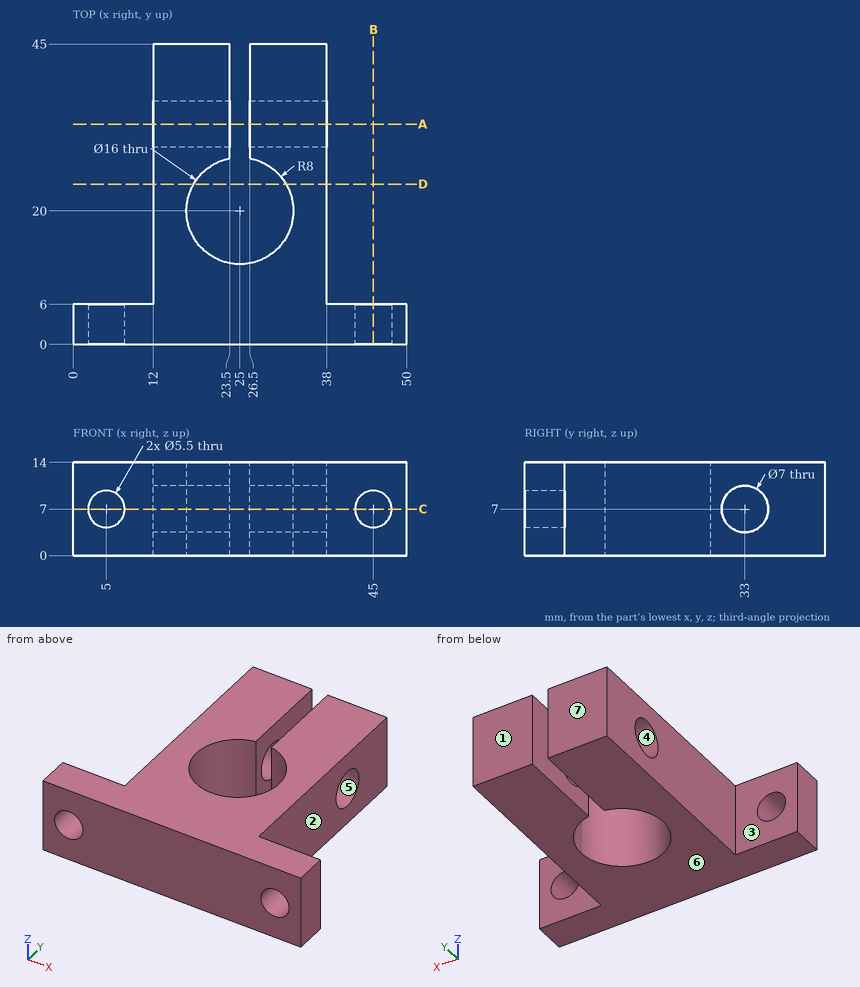
Input: dimensioned drawing with shaded views. Units: mm. Origin: part minimum x, y, z. A direction names the side the tool comes from. Give positions to 0.01 mm unless a question says otherwise; leave off trailing zeros. Write each loop counter-clockwise with the first axis right and the second up, starting at its lowest first coordinate (ties: lowest second). Pieces come first, ordered by that corner, then holes. Notation, with made-up numbers: (-36, -1) -> (10, -1) arc R24 cw to (10, 31) -> close; hole circle Ø4 at (18.5, 33.25). An arc over 180 degrees is marked (long way). Answer as a JSON object with one key per item and string values.
1. Cut plane C-C on z = 7. Output: boundary loops of the cut face in (x, y).
Ans:
{"outline": "(0, 0) -> (2.25, 0) -> (2.25, 6) -> (0, 6) -> close; (7.75, 0) -> (42.25, 0) -> (42.25, 6) -> (38, 6) -> (38, 29.5) -> (26.5, 29.5) -> (26.5, 27.86) arc R8 cw (long way) to (23.5, 27.86) -> (23.5, 29.5) -> (12, 29.5) -> (12, 6) -> (7.75, 6) -> close; (12, 36.5) -> (23.5, 36.5) -> (23.5, 45) -> (12, 45) -> close; (26.5, 36.5) -> (38, 36.5) -> (38, 45) -> (26.5, 45) -> close; (47.75, 0) -> (50, 0) -> (50, 6) -> (47.75, 6) -> close"}
2. Cut plane A-A on y = 33. Output: boundary loops of the cut face in (x, z).
Ans:
{"outline": "(12, 0) -> (23.5, 0) -> (23.5, 3.5) -> (12, 3.5) -> close; (12, 10.5) -> (23.5, 10.5) -> (23.5, 14) -> (12, 14) -> close; (26.5, 0) -> (38, 0) -> (38, 3.5) -> (26.5, 3.5) -> close; (26.5, 10.5) -> (38, 10.5) -> (38, 14) -> (26.5, 14) -> close"}
3. Contact query for flat-ended pins moving along their axis: pin 1 (6 mm diameter, centred on y = 19.5, z = 3, fed in from -X); pin 2 (1.5 mm diameter, centred on y = 15.5, z = 1.5, fed in from +X); pin 3 (6 mm diameter, centred on x = 8, z = 7.5, fed in from +Y). Output: stop coordinate, or through.
Ans:
{"pin 1": "stops at x = 12", "pin 2": "stops at x = 38", "pin 3": "stops at y = 6"}
4. Ray query, probe 1 along Y at (x, z) = (2, 8.5); probe 2 along Y at (x, z) = (15, 7.5); probe 3 along Z at (x, y) = (18.5, 33). Return the intervals inside material, ascending. Write a range as from..to.
Ans:
{"probe 1": "y = 0..6", "probe 2": "y = 0..29.54, 36.46..45", "probe 3": "z = 0..3.5, 10.5..14"}
5. Cut plane B-B on x = 45. Output: boundary loops of the cut face in (y, z), and give its area (3 significant figures).
Ans:
{"outline": "(0, 0) -> (6, 0) -> (6, 4.25) -> (0, 4.25) -> close; (0, 9.75) -> (6, 9.75) -> (6, 14) -> (0, 14) -> close", "area": "51.0 mm^2"}
6. Mould query, pull axis Y, two halves, no side actions, for the marked faces 4, 5, 6 and 7. Classes: pulls with the +Y half, pulls with the -Y half, needs draft (parallel to the pull), parting line crosses it, or undercut.
Ans:
{"face 4": "undercut", "face 5": "undercut", "face 6": "needs draft", "face 7": "pulls with the +Y half"}
7. Access query for the marked faces 1, 2 and 3. Directions: +Z, -Z, +X, -X, +Y, -Y. A direction counts if a zero-diameter tool reaches every point of the face in a straight line with its end or side. Return the directions, or none.
Ans:
{"face 1": "+Z, -Z, +X, -X, +Y", "face 2": "+Z, -Z, +X, +Y", "face 3": "+Z, -Z, -X, +Y"}
8. Cut plane D-D on y = 24. Output: boundary loops of the cut face in (x, z), and give its area (3 significant figures).
Ans:
{"outline": "(12, 0) -> (18.07, 0) -> (18.07, 14) -> (12, 14) -> close; (31.93, 0) -> (38, 0) -> (38, 14) -> (31.93, 14) -> close", "area": "170 mm^2"}
